Input: part model. Units: mm. Frame: model coordinates. A direction names the side the tool comes from. Coordinates: 2 decimals unless noted, no trailing zeros. Order: outer loops, then holes, each group sorted by start corner. A loop starts at its lowest first (then second) coordinate and runs counter-clockwise, first axis right, second up. Notation, with made-up numbers: (37, 0.5) -> (42, 0.5) arc R11 ccw to (42, 10.5) -> close; hole circle Ø4 at (-0.75, -34.75). An arc over 180 degrees is marked (long way). Use one line per item in the form item = value. Start each with the question number.
1) Section query B-B on y = 27.5. Output: boundary loops of the cut face in (x, z), then the cut area to 3 significant figures.
2) Section query A-A on y = -11. Output: boundary loops of the cut face in (x, z), then the cut area to 3 significant figures.
3) Access query for faces 1 (the flat face through (-8.707, 18.123, -1.987)), 2 (the flat face through (1, 10, 1)), 3 (the flat face through (-18.104, 19.72, -5.407)), 4 (the flat face through (19.627, 19.72, 7.879)), 5 (the flat face through (10.087, 18.123, 4.853)). Directions: +Z, -Z, +X, -X, +Y, -Y. A direction counts if a zero-diameter tool reaches every point of the face in a straight line with its end or side. Return the directions, or none.
4) Pin query (flat end, axial travel): pin 1 (10 mm diameter, centred on y = 32, z = 11, fed in from +X); pin 2 (1.5 mm diameter, centred on x = 20, z = -5, fed in from +Y); pin 3 (1.5 mm diameter, centred on x = 9.5, y = 2, fed in from -Z). Return the tip coordinate at first contact, or that it passes through.
5) Section query D-D on y = 35.5. Output: boundary loops of the cut face in (x, z).
6) Section query C-C on x = -33. Output: boundary loops of the cut face in (y, z).
7) Draft query along X for faces 6 (the flat face through (30, -18, 2)), 7 (the flat face through (-35, -25, -2)), 8 (the flat face through (31.69, -9.55, -20.38)). Return one class per face: pulls with the +X half, pulls with the -X half, needs draft (parallel to the pull), parting line crosses it, or undercut.
8) Ray query, line 1 along X through (y, z) = (-13, -3.5); line 2 along Y through (x, z) = (2, -13); line 3 along Y through (x, z) = (-35.5, -17). Return the intervals inside material, ascending.
from build123d import *

# Parameters (mm, degrees)
EXTRUDE_1_DEPTH     = 25
SKETCH_2_W          = 60
SKETCH_2_H          = 15
CUT_EXTRUDE_1_DEPTH = 69.738635424
EXTRUDE_2_DEPTH     = 40
SKETCH_4_R          = 5
CUT_EXTRUDE_2_DEPTH = 79.882076454
SKETCH_5_W          = 20
SKETCH_5_H          = 30
CUT_EXTRUDE_3_DEPTH = 40


with BuildPart() as part:
    # Эскиз1 → Бобышка-Вытянуть1 (new body)
    with BuildSketch(Plane(origin=(0, 0, 0), x_dir=(1, 0, 0), z_dir=(0, 1, 0))):
        Polygon((-40, 25), (19, 25), (40, 17.35662508), (40, -25), (-19, -25), (-40, -17.35662508), align=None)
    extrude(amount=-EXTRUDE_1_DEPTH)

    # Эскиз2 → Вырез-Вытянуть1 (cut, through all)
    with BuildSketch(Plane.XY.offset(25)):
        with Locations((0, -17.5)):
            Rectangle(SKETCH_2_W, SKETCH_2_H)
    extrude(amount=-CUT_EXTRUDE_1_DEPTH, mode=Mode.SUBTRACT)

    # Эскиз3 → Бобышка-Вытянуть2 (add)
    with BuildSketch(Plane(origin=(0, 0, 0), x_dir=(1, 0, 0), z_dir=(0, 1, 0))):
        Polygon((-12.902085739, 19.7), (24.685619092, 6.019194267), (14.425014792, -22.171584357), (-23.162690039, -8.490778624), align=None)
    extrude(amount=EXTRUDE_2_DEPTH)

    # Эскиз4 → Вырез-Вытянуть2 (cut, through all)
    with BuildSketch(Plane(origin=(19.863418464, 0, 7.229693072), x_dir=(0.34202014332567277, 0, -0.939692620785907), z_dir=(0.939692620785907, 0, 0.34202014332567277))):
        with BuildLine():
            Line((-15.900828584, 40), (-15.900828584, 25))
            ThreePointArc((-15.900828584, 25), (-11.507430302, 35.606601718), (-0.900828584, 40))
            Line((-0.900828584, 40), (-15.900828584, 40))
        make_face()
        with BuildLine():
            Line((14.099171416, 40), (-0.900828584, 40))
            ThreePointArc((-0.900828584, 40), (9.705773134, 35.606601718), (14.099171416, 25))
            Line((14.099171416, 25), (14.099171416, 40))
        make_face()
        with Locations((-0.900828584, 25)):
            Circle(SKETCH_4_R)
    extrude(amount=-CUT_EXTRUDE_2_DEPTH, mode=Mode.SUBTRACT)

    # Эскиз5 → Вырез-Вытянуть3 (cut)
    with BuildSketch(Plane(origin=(-5.438403671, 0, 14.941891285), x_dir=(0.9396926207859105, 0, 0.34202014332566305), z_dir=(-0.34202014332566305, 0, 0.9396926207859105))):
        with Locations((1.138208415, 25)):
            Rectangle(SKETCH_5_W, SKETCH_5_H)
    extrude(amount=-CUT_EXTRUDE_3_DEPTH, mode=Mode.SUBTRACT)


solid = part.part
Answers below:
q1.outline = (-23.09, 8.29) -> (-19.51, -1.54) -> (-10.12, 1.88) -> (-13.69, 11.71) -> close; (-16.55, -9.67) -> (-12.97, -19.5) -> (-3.58, -16.08) -> (-7.15, -6.25) -> close; (5.1, 18.55) -> (8.68, 8.72) -> (18.07, 12.15) -> (14.5, 21.97) -> close; (11.64, 0.59) -> (15.22, -9.24) -> (24.61, -5.82) -> (21.04, 4.01) -> close
q1.area = 418 mm^2
q2.outline = (-40, -25) -> (-30, -25) -> (-30, 21) -> (-40, 17.36) -> close; (30, -21) -> (40, -17.36) -> (40, 25) -> (30, 25) -> close
q2.area = 884 mm^2
q3.face_1 = +Z, +Y
q3.face_2 = +Y
q3.face_3 = -Z, -X, +Y
q3.face_4 = +Z, +X, +Y
q3.face_5 = -Z, +Y
q4.pin_1 = 20.31
q4.pin_2 = 34.4
q4.pin_3 = -11.82
q5.outline = (-21.7, 4.46) -> (-14.37, -15.67) -> (-4.97, -12.25) -> (-12.3, 7.88) -> close; (6.49, 14.72) -> (13.82, -5.41) -> (23.22, -1.99) -> (15.89, 18.14) -> close
q6.outline = (-25, -25) -> (0, -25) -> (0, 19.9) -> (-25, 19.9) -> close
q7.face_6 = undercut
q7.face_7 = needs draft
q7.face_8 = pulls with the +X half
q8.line_1 = -40 to -30, 30 to 40
q8.line_2 = -10 to 10
q8.line_3 = -25 to 0
